Could you check a few things on this model? Use its own coordinates, in mm. A direction names the side the tool comes from. Coordinates: 2 decimals unless noted, no trailing zeros. Loops run counter-clockwise (first coordinate to the right, second up) from the corner with the lowest first, then second, coordinate; pieces in that order, holes last.
1) For faces 1 (the face through (32, -13, 9.479)), 2 (the face through (19, -13, 3.129)), which set-ups out of +Z, -Z, +X, -X, +Y, -Y let a thin tool reach every point of the face, with its end or its side?
2) Imagine slicing it at B-B on x = 31. Please give me the cut outline in (y, z).
3) Imagine slicing it at C-C on z = 22. Please give me the cut outline in (x, y), plus the area to 3 significant figures.
4) Imagine slicing it at A-A on y = -11.25. Please give me the cut outline in (x, z).
5) If I drill on line 1 along Z through (x, y) = (37, -1.5); line 2 along X through (y, z) = (-23, 6.5); line 3 along X through (y, z) = (-12, 7.5), over which ranges is the centre line in solid material (lowest first)?
6) Will these pins go through, and if not, where does the flat tip stop? P1, Ø1.9, axis at y = -8.5, z = 5.5, coming from the +X side; P2, Ø5, axis at y = -10.5, z = 6, coming from the -X side; P3, Ø10, axis at x = 34.5, z = 7, coming from the -Y side; P4, Ø5, axis at y = -9, z = 27, coming from the -X side.
7) Thinking about a two-plate mould opening in X: for faces 3 (the face through (25.84, -13, 6)), 4 (the face through (44.8, -12.52, 19.23)), 5 (the face through (38.54, -13, 6)), 6 (the face through (19.4, -12.52, 18.87)), which applies, released by +X, released by -X, zero draft, split by the parting line, or undercut?
```python
from build123d import *

# Parameters (mm, degrees)
F0_W     = 38.1
F0_H     = 31.75
F1_DEPTH = 25.4
F3_DEPTH = 25.4
F5_DEPTH = 25.4
F6_W     = 12.7
F6_H     = 6.35
F7_DEPTH = 25.4


with BuildPart() as f1:
    # F0 (on Front) → F1 (new body)
    with BuildSketch(Plane.XZ):
        with Locations((32.189709, 19.003802)):
            Rectangle(F0_W, F0_H)
    extrude(amount=F1_DEPTH)

    # F2 (on Front) → F3 (cut)
    with BuildSketch(Plane.XZ):
        Polygon((51.239709, 34.878802), (38.539709, 34.878802), (51.239709, 3.128802), align=None)
    extrude(amount=F3_DEPTH, mode=Mode.SUBTRACT)

    # F4 (on Front) → F5 (cut)
    with BuildSketch(Plane.XZ):
        Polygon((13.139709, 3.309423), (25.839709, 34.878802), (13.139709, 35.059423), align=None)
    extrude(amount=F5_DEPTH, mode=Mode.SUBTRACT)

    # F6 (on Front) → F7 (cut)
    with BuildSketch(Plane.XZ):
        with Locations((32.189709, 6.303802)):
            Rectangle(F6_W, F6_H)
    extrude(amount=F7_DEPTH, mode=Mode.SUBTRACT)


solid = f1.part
```
Filled in:
1. face 1: -Z, +Y, -Y
1. face 2: -Z, +X, -X, +Y, -Y
2. outline: (-25.4, 9.48) - (0, 9.48) - (0, 34.88) - (-25.4, 34.88) - close
3. outline: (20.66, -25.4) - (43.69, -25.4) - (43.69, 0) - (20.66, 0) - close
3. area: 585 mm2
4. outline: (13.14, 3.13) - (25.84, 3.13) - (25.84, 9.48) - (38.54, 9.48) - (38.54, 3.13) - (51.24, 3.13) - (38.54, 34.88) - (25.84, 34.88) - (13.14, 3.31) - close
5. line 1: z = 9.48 to 34.88
5. line 2: x = 14.42 to 25.84, 38.54 to 49.89
5. line 3: x = 14.83 to 25.84, 38.54 to 49.49
6. P1: stops at x = 50.67
6. P2: stops at x = 13.22
6. P3: stops at y = -25.4
6. P4: stops at x = 21.66
7. face 3: undercut
7. face 4: released by +X
7. face 5: undercut
7. face 6: released by -X
